Check sheet for the modelled part. Datum: model origin and axes. Units: mm. Coordinates: 2 decimals unless noted, no trailing zeros. Write each loop counter-clockwise with the first axis right and the second up, starting at its lowest first coordinate (ties: lowest second). Pieces come first, ordered by that corner, then holes. Notation, with made-up numbers: (76, -12.75) -> (130, -12.75) arc R20 ccw to (130, -5.75) -> close; hole circle Ø7 at (0, 42.5). An arc over 180 degrees is marked (long way). Put each result on its own line as item: value.
```python
from build123d import *

# Parameters (mm, degrees)
SKETCH1_R           = 20
SKETCH1_R_2         = 7.5
BOSS_EXTRUDE1_DEPTH = 2
CUT_EXTRUDE1_REACH  = 140.669
SKETCH3_R           = 2


with BuildPart() as part:
    # Sketch1 → Boss-Extrude1 (new body)
    # profile 1 of 2: a face of its own
    with BuildSketch(Plane.XY):
        with BuildLine():
            ThreePointArc((-60, 0), (-52.867640737, 28.372743309), (-33.166247904, 50))
            Line((-33.166247904, 50), (-60, 50))
            Line((-60, 50), (-60, 0))
        make_face()
    # profile 2 of 2: a face of its own
    with BuildSketch(Plane.XY):
        with BuildLine():
            Line((117.67766953, 17.32233047), (70.010033914, -30.345305145))
            Line((70.010033914, -30.345305145), (51.7606265, -30.345305145))
            ThreePointArc((51.7606265, -30.345305145), (-52.061109807, -29.826847732), (0, 60))
            Line((0, 60), (100, 60))
            ThreePointArc((100, 60), (123.096988313, 44.567085809), (117.67766953, 17.32233047))
        make_face()
        with Locations((100, 35)):
            Circle(SKETCH1_R, mode=Mode.SUBTRACT)
        Circle(SKETCH1_R_2, mode=Mode.SUBTRACT)
    extrude(amount=BOSS_EXTRUDE1_DEPTH)

    # Sketch3 → Cut-Extrude1 (cut, up to next)
    with BuildSketch(Plane.XY.offset(2), mode=Mode.PRIVATE) as cut_extrude1_sk1:
        with Locations((50, 50)):
            Circle(SKETCH3_R)
    cut_extrude1_tool1 = extrude(cut_extrude1_sk1.sketch, amount=-CUT_EXTRUDE1_REACH, mode=Mode.PRIVATE) & part.part
    # Sketch3 → Cut-Extrude1 (cut, up to next)
    with BuildSketch(Plane.XY.offset(2), mode=Mode.PRIVATE) as cut_extrude1_sk2:
        with Locations((70, 9.654694855)):
            Circle(SKETCH3_R)
    cut_extrude1_tool2 = extrude(cut_extrude1_sk2.sketch, amount=-CUT_EXTRUDE1_REACH, mode=Mode.PRIVATE) & part.part
    add(cut_extrude1_tool1.solids().sort_by_distance((50, 50, 2))[0], mode=Mode.SUBTRACT)
    add(cut_extrude1_tool2.solids().sort_by_distance((70, 9.654695, 2))[0], mode=Mode.SUBTRACT)


solid = part.part
```
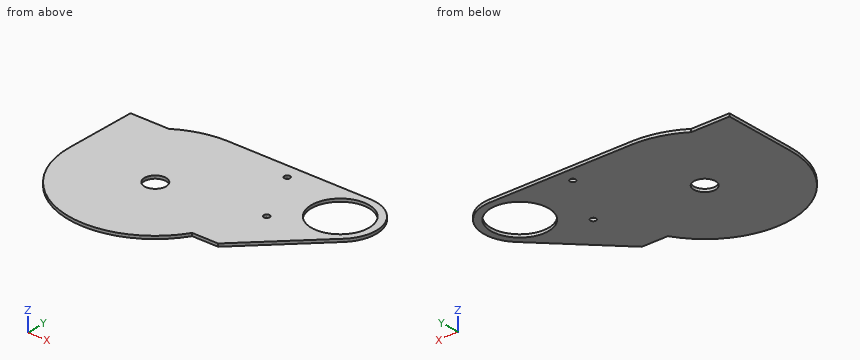
Q1. Cross-section at D-D (y = -14). Record the cut outline in (x, z), plus the area to 3 significant figures.
Recorded:
outline: (-58.34, 0) -> (86.36, 0) -> (86.36, 2) -> (-58.34, 2) -> close
area: 289 mm2
Q2. Cross-section at C-C (z = 1.4). Record the cut outline in (x, y), plus the area to 3 significant figures.
Recorded:
outline: (-60, 0) arc R60 ccw to (51.76, -30.35) -> (70.01, -30.35) -> (117.68, 17.32) arc R25 ccw to (100, 60) -> (0, 60) arc R60 ccw to (-33.17, 50) -> (-60, 50) -> close; hole circle Ø15 at (0, 0); hole circle Ø4 at (50, 50); hole circle Ø4 at (70, 9.65); hole circle Ø40 at (100, 35)
area: 15,300 mm2
Q3. Cross-section at B-B (x = 83). Record the cut outline in (y, z).
Recorded:
outline: (-17.36, 0) -> (24.46, 0) -> (24.46, 2) -> (-17.36, 2) -> close; (45.54, 0) -> (60, 0) -> (60, 2) -> (45.54, 2) -> close
Q4. Cross-section at A-A (y = 35). Record the cut outline in (x, z).
Recorded:
outline: (-60, 0) -> (80, 0) -> (80, 2) -> (-60, 2) -> close; (120, 0) -> (125, 0) -> (125, 2) -> (120, 2) -> close
Q5. Material ranges on line 1 along Y through (x, z) = (70, 1.35); line 2 along X through (y, z) = (50.5, 0.15); line 3 along Y through (x, z) = (101.5, 1.9), recorded low to high.
Recorded:
line 1: y = -30.35 to 7.65, 11.65 to 60
line 2: x = -32.4 to 48.06, 51.94 to 87.36, 112.64 to 119.62
line 3: y = 1.14 to 15.06, 54.94 to 59.95
Q6. Depth check by flat-ended pin: P1, Ø2.5, axis at x = 50, y = 50, coming from the -Z side; P2, Ø0.6, axis at x = 57, z = 0.5, coming from the -Y side. Enter the tip coordinate at first touch or a pass-through.
Recorded:
P1: passes through
P2: stops at y = -30.35
